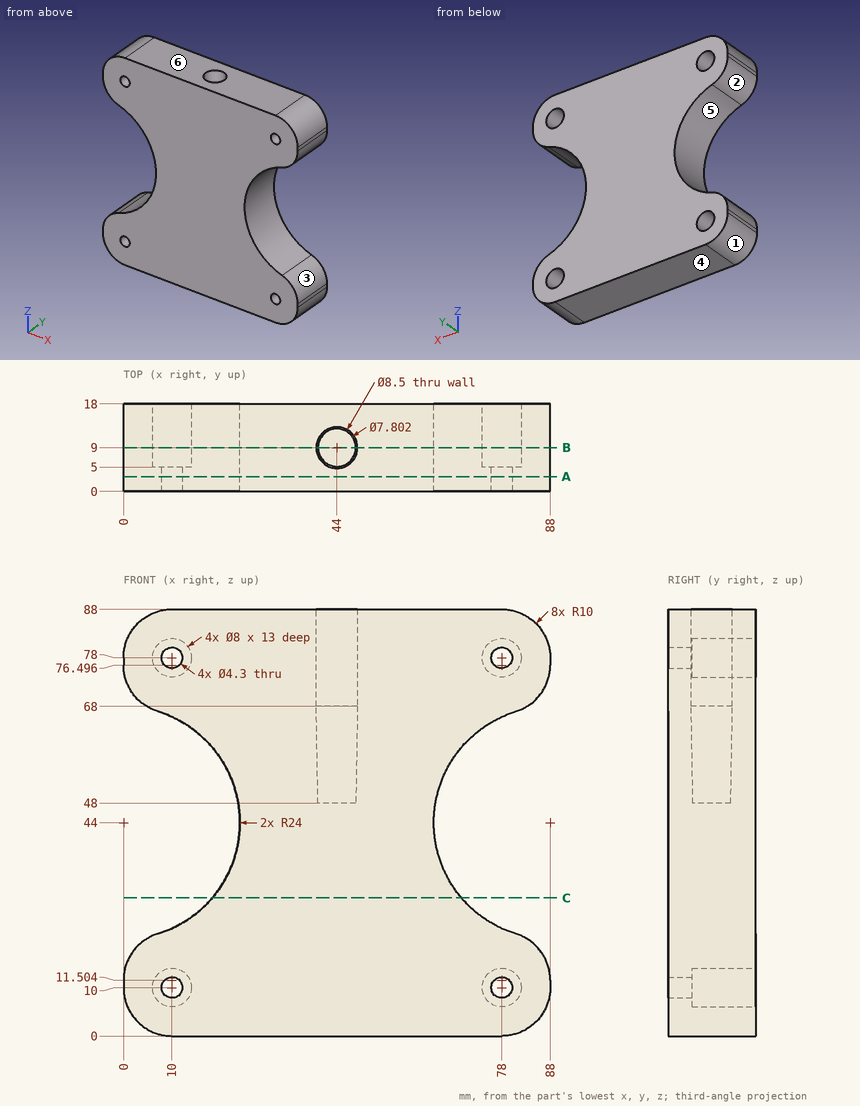
Geometry: see drawing. Coordinates: mm, zero at the bounding-box minimum. A direction names the side the tool comes from. Give positions to 0.01 mm unless a question says otherwise; leave off trailing zeros. Order: outer loops, then holes, each group sorted by start corner. A loop starts at its lowest first (then second) coordinate and runs counter-clockwise, first axis right, second up. Notation, with made-up numbers: (-37.5, 27.5) - (-14.5, 27.5) arc R29 ccw to (-14.5, 57.5) - close; hole circle Ø4 at (37.5, 30.5). An arc over 180 degrees is marked (long way). Use a Markdown table: item, result.
(1) Section query C-C (z = 28.5). Output: boundary loops of the cut face in (x, y).
Computed values:
| item | result |
|---|---|
| outline | (18.32, 0) - (69.68, 0) - (69.68, 18) - (18.32, 18) - close |
(2) Section query A-A (y = 3). Output: boundary loops of the cut face in (x, z), then the cut area to 3 significant figures.
Computed values:
| item | result |
|---|---|
| outline | (0, 10) arc R10 ccw to (10, 0) - (78, 0) arc R10 ccw to (88, 10) - (88, 11.5) arc R10 ccw to (80.94, 21.06) arc R24 cw to (80.94, 66.94) arc R10 ccw to (88, 76.5) - (88, 78) arc R10 ccw to (78, 88) - (10, 88) arc R10 ccw to (0, 78) - (0, 76.5) arc R10 ccw to (7.06, 66.94) arc R24 cw to (7.06, 21.06) arc R10 ccw to (0, 11.5) - close; hole circle Ø4.3 at (10, 10); hole circle Ø4.3 at (10, 78); hole circle Ø4.3 at (78, 10); hole circle Ø4.3 at (78, 78) |
| area | 5,740 mm2 |
(3) Access query for the marked faces 1, 2 and 3. Directions: +Z, -Z, +X, -X, +Y, -Y. A direction counts if a zero-diameter tool reaches every point of the face in a straight line with its end or side. Return the directions, or none.
Computed values:
| item | result |
|---|---|
| face 1 | -Z, -X, +Y, -Y |
| face 2 | -X, +Y, -Y |
| face 3 | +X, +Y, -Y |
(4) Section query B-B (y = 9). State how many separate pieces and enclosed holes the cut face has, then the cut area to 3 significant figures.
Computed values:
| item | result |
|---|---|
| separate pieces | 1 |
| enclosed holes | 4 |
| area | 5,260 mm2 |
(5) Draft query along Z for the marked faces 4, 5 and 6. Return one class per face: released by +Z, released by -Z, zero draft, split by the parting line, or undercut.
Computed values:
| item | result |
|---|---|
| face 4 | released by -Z |
| face 5 | undercut |
| face 6 | released by +Z |
(6) Pin query (flat end, axial travel): pin 1 (3 mm diameter, centred on y = 8, z = 68.5, fed in from +X); pin 2 (5 mm diameter, centred on x = 78, z = 78, fed in from +Y); pin 3 (2 mm diameter, centred on y = 6.5, z = 73, fed in from +X). Return the tip coordinate at first contact, or that it passes through.
Computed values:
| item | result |
|---|---|
| pin 1 | stops at x = 85.6 |
| pin 2 | stops at y = 5 |
| pin 3 | stops at x = 87.68 |
(7) Line query: line 1 (X direction, y = 14, z = 10); line 2 (X direction, y = 3.3, z = 10); line 3 (Y direction, x = 44, z = 82.5). Output: solid intervals per line, ascending. Write a range as from..to.
Computed values:
| item | result |
|---|---|
| line 1 | x = 0..6, 14..74, 82..88 |
| line 2 | x = 0..7.85, 12.15..75.85, 80.15..88 |
| line 3 | y = 0..4.75, 13.25..18 |
